from build123d import *

# Parameters (mm, degrees)
EXTRUDE_1_DEPTH         = 24
SKETCH_2_W              = 20.4
SKETCH_2_H              = 6.8
CUT_EXTRUDE_1_DEPTH     = 21
CUT_EXTRUDE_2_REACH     = 36.86
SKETCH_3_W              = 12.046070068
SKETCH_3_H              = 8.16612352
FILLET_1_R              = 1
CUT_EXTRUDE_START       = -10.5
CUT_EXTRUDE_3_OUTLINE_R = 6.75
CUT_EXTRUDE_3_DEPTH     = 2.8
CUT_EXTRUDE_START_2     = -7.7
CUT_EXTRUDE_4_OUTLINE_R = 5
CUT_EXTRUDE_4_DEPTH     = 0.9


# Read off the part's stored shape, not the designer's step: the extrude step, the extrude step
with BuildPart() as part:
    # Sketch 3D_1 → Extrude 1 (new body)
    with BuildSketch(Plane(origin=(0, 0, 0), x_dir=(0, 0.909688003863034, -0.41529234958964595), z_dir=(1, 0, 0))):
        Polygon((0, 0), (20.922824089, 9.551724041), (25.28339376, 0), (4.360569671, -9.551724041), align=None)
    extrude(amount=EXTRUDE_1_DEPTH)

    # Sketch 2 → Cut-Extrude 1 (cut)
    with BuildSketch(Plane(origin=(0, 23, 0), x_dir=(1, 0, 0), z_dir=(0, 1, 0))):
        with Locations((12, 3.4)):
            Rectangle(SKETCH_2_W, SKETCH_2_H)
    extrude(amount=-CUT_EXTRUDE_1_DEPTH, mode=Mode.SUBTRACT)

    # Sketch 3 → Cut-Extrude 2 (cut, up to next)
    with BuildSketch(Plane.XZ, mode=Mode.PRIVATE) as cut_extrude_2_sk1:
        with Locations((12, 0)):
            Rectangle(SKETCH_3_W, SKETCH_3_H)
    cut_extrude_2_tool1 = extrude(cut_extrude_2_sk1.sketch, amount=-CUT_EXTRUDE_2_REACH, mode=Mode.PRIVATE) & part.part
    add(cut_extrude_2_tool1.solids().sort_by_distance((12, 0, 0))[0], mode=Mode.SUBTRACT)

    # Fillet 1
    fillet_1_edges = [part.edges().sort_by_distance(p)[0] for p in [
        (24, 23, -5.25),
        (24, 0, -5.25),
        (24, 11.5, -10.5),
        (12, 0, -10.5),
        (0, 0, -5.25),
        (0, 11.5, -10.5),
        (12, 23, -10.5),
        (0, 23, -5.25),
    ]]
    fillet(fillet_1_edges, radius=FILLET_1_R)

    # Cut-Extrude 3 outline → Cut-Extrude 3 (cut)
    with BuildSketch(Plane.XY.offset(CUT_EXTRUDE_START)):
        with Locations((12, 11.3)):
            Circle(CUT_EXTRUDE_3_OUTLINE_R)
    extrude(amount=CUT_EXTRUDE_3_DEPTH, mode=Mode.SUBTRACT)

    # Cut-Extrude 4 outline → Cut-Extrude 4 (cut)
    with BuildSketch(Plane.XY.offset(CUT_EXTRUDE_START_2)):
        with Locations((12, 11.3)):
            Circle(CUT_EXTRUDE_4_OUTLINE_R)
    extrude(amount=CUT_EXTRUDE_4_DEPTH, mode=Mode.SUBTRACT)


solid = part.part
Design review of the part built by this model. Coordinates are the model's own, in mm. A direction names the side the tool comes from. Round coordinates to 2 decimals unless told otherwise and drop trailing zeros. Loops run counter-clockwise (first coordinate to the right, second up) from the corner with the lowest first, then second, coordinate; pieces in that order, holes last. Notation, with made-up numbers: (68, 28.5) -> (111, 28.5) arc R32 ccw to (111, 54.5) -> close; hole circle Ø7 at (-5.75, 63.25). An arc over 180 degrees is marked (long way). Use one line per item in the form item = value. Start each with the question number.
Q1. We need section C-C on x = 12. Give the boundary of the cut face in (y, z).
Q2. For pin 1 Ø1.6 at (x, y) = (11, 1) entering from +Z; pin 2 Ø13 at (x, y) = (12, 11.3) entering from +Z; pin 3 Ø8 at (x, y) = (3, 14.5) entering from +Z, all flat-tipped, find the tip position at first contact; note any pin that passes through.
Q3. Machinability: for faces 4 (the face through (5.977, 1, -2)), 5 (the face through (23.699, 0.285, -4.684)), 6 (the face through (12, 2, -5)), which of the approach directions +Z, -Z, +X, -X, +Y, -Y give a long, thin tool a straight path to every point of the face, cutting with its end or side? Answer none if there is none.
Q4. We need section D-D on x = 21. Give the boundary of the cut face in (y, z).
Q5. We need section B-B on z = -3.75. Give the boundary of the cut face in (x, y).
Q6. Wall thickness on line 1 along X through (y, z) = (5.75, -1.25); line 2 along X through (y, z) = (1, -0.5); line 3 along Y through (x, z) = (12, -7.45): over which ranges is each line inside the solid? List them lowest first. Write a range as [from, to].
Q7. Draft analysis for pull direction Y (two halves, no side actions). For faces 1 (the face through (18.438, 13.328, -9.12)), 2 (the face through (0.285, 11.353, -10.199)), 3 (the face through (12.154, 22.715, -10.199)), state which applies: +Y half, -Y half, draft (parallel to the pull), parting line (faces both ways), or undercut.
Q8. We need section A-A on y = 11.3. Give the boundary of the cut face in (x, z), then the cut area to 3 significant figures.
Calculated:
q1.outline = (0, -9.5) arc R1 ccw to (1, -10.5) -> (4.55, -10.5) -> (4.55, -7.7) -> (6.3, -7.7) -> (6.3, -6.8) -> (2, -6.8) -> (2, -4.08) -> (0, -4.08) -> close; (16.3, -7.7) -> (18.05, -7.7) -> (18.05, -10.5) -> (22, -10.5) arc R1 ccw to (23, -9.5) -> (23, -6.8) -> (16.3, -6.8) -> close
q2.pin_1 = -4.08
q2.pin_2 = -6.8
q2.pin_3 = 0
q3.face_4 = +Z, +Y, -Y
q3.face_5 = +Z, -Z, +X, -Y
q3.face_6 = +Z, +Y
q4.outline = (0, -9.5) arc R1 ccw to (1, -10.5) -> (22, -10.5) arc R1 ccw to (23, -9.5) -> (23, -6.8) -> (2, -6.8) -> (2, 0) -> (0, 0) -> close
q5.outline = (0, 1) arc R1 ccw to (1, 0) -> (5.98, 0) -> (5.98, 2) -> (1.8, 2) -> (1.8, 23) -> (1, 23) arc R1 ccw to (0, 22) -> close; (18.02, 0) -> (23, 0) arc R1 ccw to (24, 1) -> (24, 22) arc R1 ccw to (23, 23) -> (22.2, 23) -> (22.2, 2) -> (18.02, 2) -> close
q6.line_1 = [0, 1.8], [22.2, 24]
q6.line_2 = [0, 5.98], [18.02, 24]
q6.line_3 = [0, 6.3], [16.3, 23]
q7.face_1 = undercut
q7.face_2 = draft
q7.face_3 = +Y half
q8.outline = (0, -9.5) arc R1 ccw to (1, -10.5) -> (5.25, -10.5) -> (5.25, -7.7) -> (7, -7.7) -> (7, -6.8) -> (1.8, -6.8) -> (1.8, 0) -> (0, 0) -> close; (17, -7.7) -> (18.75, -7.7) -> (18.75, -10.5) -> (23, -10.5) arc R1 ccw to (24, -9.5) -> (24, 0) -> (22.2, 0) -> (22.2, -6.8) -> (17, -6.8) -> close
q8.area = 66.1 mm²
